Can you work these out from the model? Positions are in its coordinate system, mm. A direction names the side the tool comes from. Give positions to 0.01 mm unless a question says otherwise; leave off trailing zeros. Loops run counter-clockwise (first coordinate to the right, second up) from the corner with the lowest first, then second, coordinate; pieces in that order, holes last. Notation, with made-up numbers: (25.25, 80) - (51.25, 80) arc R24 cw to (51.25, 95) - close; hole circle Ø6 at (-4, -37.75). An arc over 180 degrees is marked (long way). Answer in a Markdown table with one row per item.
from build123d import *

# Parameters (mm, degrees)
SKETCH_1_W                       = 50
SKETCH_1_H                       = 20
SM_BASE_FLANGE_1_DEPTH           = 2
SM_EDGE_FLANGE_1_STRIP_W         = 9.4732
SM_EDGE_FLANGE_1_STRIP_H         = 2
SM_EDGE_FLANGE_1_STRIP_CUT_DEPTH = 20
SM_EDGE_FLANGE_1_DEPTH           = 20
SM_EDGE_FLANGE_2_STRIP_W         = 9.4732
SM_EDGE_FLANGE_2_STRIP_H         = 2
SM_EDGE_FLANGE_2_STRIP_CUT_DEPTH = 20
SM_EDGE_FLANGE_2_DEPTH           = 20
SKETCH_12_R                      = 2
CUT_EXTRUDE_1_DEPTH              = 2
CUT_EXTRUDE_2_REACH              = 61.372
SKETCH_13_R                      = 2


# Sheet-metal steps are written as plain solids
with BuildPart() as part:
    # Sketch 1 → Базовая кромка1 (new body)
    with BuildSketch(Plane(origin=(0, 0, 0), x_dir=(1, 0, 0), z_dir=(0, 1, 0))):
        with Locations((25, 10)):
            Rectangle(SKETCH_1_W, SKETCH_1_H)
    extrude(amount=-SM_BASE_FLANGE_1_DEPTH)

    # Ребро-кромка1 strip (across the edge) → Ребро-кромка1 strip cut (cut)
    with BuildSketch(Plane(origin=(50, 0, 0), x_dir=(-1, 0, 0), z_dir=(0, 0, -1))):
        with Locations((-2, -1)):
            Rectangle(SM_EDGE_FLANGE_1_STRIP_W, SM_EDGE_FLANGE_1_STRIP_H)
    extrude(amount=SM_EDGE_FLANGE_1_STRIP_CUT_DEPTH, mode=Mode.SUBTRACT)

    # Ребро-кромка1 section (across the edge) → Ребро-кромка1 (add)
    with BuildSketch(Plane(origin=(50, 0, 0), x_dir=(-1, 0, 0), z_dir=(0, 0, -1))):
        with BuildLine():
            Line((0, 0.7366), (0, 25))
            Line((0, 25), (2, 25))
            Line((2, 25), (2, 0.7366))
            ThreePointArc((2, 0.7366), (2.215745145, 0.215745145), (2.7366, 0))
            Line((2.7366, 0), (2.7366, -2))
            ThreePointArc((2.7366, -2), (0.801531583, -1.198468417), (0, 0.7366))
        make_face()
    extrude(amount=SM_EDGE_FLANGE_1_DEPTH)

    # Ребро-кромка2 strip (across the edge) → Ребро-кромка2 strip cut (cut)
    with BuildSketch(Plane.XY.offset(-20)):
        with Locations((-2, -1)):
            Rectangle(SM_EDGE_FLANGE_2_STRIP_W, SM_EDGE_FLANGE_2_STRIP_H)
    extrude(amount=SM_EDGE_FLANGE_2_STRIP_CUT_DEPTH, mode=Mode.SUBTRACT)

    # Ребро-кромка2 section (across the edge) → Ребро-кромка2 (add)
    with BuildSketch(Plane.XY.offset(-20)):
        with BuildLine():
            Line((0, 0.7366), (0, 25))
            Line((0, 25), (2, 25))
            Line((2, 25), (2, 0.7366))
            ThreePointArc((2, 0.7366), (2.215745145, 0.215745145), (2.7366, 0))
            Line((2.7366, 0), (2.7366, -2))
            ThreePointArc((2.7366, -2), (0.801531583, -1.198468417), (0, 0.7366))
        make_face()
    extrude(amount=SM_EDGE_FLANGE_2_DEPTH)

    # Эскиз12 → Вырез-Вытянуть1 (cut)
    with BuildSketch(Plane.XZ.offset(2)):
        with Locations(Location((25, -5, 0), (0, 0, 270))):
            Circle(SKETCH_12_R)
        with Locations(Location((25, -15, 0), (0, 0, 270))):
            Circle(SKETCH_12_R)
    extrude(amount=-CUT_EXTRUDE_1_DEPTH, mode=Mode.SUBTRACT)

    # Вырез-Вытянуть2: up to this face of the body (flat: up to its plane)
    cut_extrude_2_end = Plane(part.part.faces().sort_by_distance((0, 12.8683, -10))[0])
    # Эскиз13 → Вырез-Вытянуть2 (cut, up to the picked face)
    with BuildSketch(Plane(origin=(50, 0, 0), x_dir=(0, 0, -1), z_dir=(1, 0, 0)), mode=Mode.PRIVATE) as cut_extrude_2_sk1:
        with Locations(Location((10, 8, 0), (0, 0, 90))):
            Circle(SKETCH_13_R)
    cut_extrude_2_tool1 = split(extrude(cut_extrude_2_sk1.sketch, amount=-CUT_EXTRUDE_2_REACH, mode=Mode.PRIVATE), bisect_by=cut_extrude_2_end, keep=Keep.BOTH, mode=Mode.PRIVATE)
    # Эскиз13 → Вырез-Вытянуть2 (cut, up to the picked face)
    with BuildSketch(Plane(origin=(50, 0, 0), x_dir=(0, 0, -1), z_dir=(1, 0, 0)), mode=Mode.PRIVATE) as cut_extrude_2_sk2:
        with Locations(Location((10, 18, 0), (0, 0, 90))):
            Circle(SKETCH_13_R)
    cut_extrude_2_tool2 = split(extrude(cut_extrude_2_sk2.sketch, amount=-CUT_EXTRUDE_2_REACH, mode=Mode.PRIVATE), bisect_by=cut_extrude_2_end, keep=Keep.BOTH, mode=Mode.PRIVATE)
    add(cut_extrude_2_tool1.solids().sort_by(Axis((50, 8, -10), (-1, 0, 0)))[0], mode=Mode.SUBTRACT)
    add(cut_extrude_2_tool2.solids().sort_by(Axis((50, 18, -10), (-1, 0, 0)))[0], mode=Mode.SUBTRACT)


solid = part.part
Q1. Imagine slicing it at B-B, the plane z = -10. Write out the boundary of the cut face in (x, y), and give its area (3 significant figures).
Checked values:
| item | result |
|---|---|
| outline | (0, 0.74) arc R2.74 ccw to (2.74, -2) - (47.26, -2) arc R2.74 ccw to (50, 0.74) - (50, 6) - (48, 6) - (48, 0.74) arc R0.74 cw to (47.26, 0) - (2.74, 0) arc R0.74 cw to (2, 0.74) - (2, 6) - (0, 6) - close; (0, 10) - (2, 10) - (2, 16) - (0, 16) - close; (0, 20) - (2, 20) - (2, 25) - (0, 25) - close; (48, 10) - (50, 10) - (50, 16) - (48, 16) - close; (48, 20) - (50, 20) - (50, 25) - (48, 25) - close |
| area | 165 mm² |
Q2. Imagine slicing it at C-C, the plane z = -5. Write out the boundary of the cut face in (x, y).
Checked values:
| item | result |
|---|---|
| outline | (0, 0.74) arc R2.74 ccw to (2.74, -2) - (23, -2) - (23, 0) - (2.74, 0) arc R0.74 cw to (2, 0.74) - (2, 25) - (0, 25) - close; (27, -2) - (47.26, -2) arc R2.74 ccw to (50, 0.74) - (50, 25) - (48, 25) - (48, 0.74) arc R0.74 cw to (47.26, 0) - (27, 0) - close |
Q3. If we mould it in two halves opening along Z, with no side actions, what happens to faces 1 (the face through (23, -1, -15)), 2 (the face through (1.014, 16.526, -8.648)), 3 (the face through (25.1, -0.4, -20)), 4 (the face through (49.177, -1.22, -9.86))? For each: released by +Z, released by -Z, zero draft, split by the parting line, or undercut.
Checked values:
| item | result |
|---|---|
| face 1 | undercut |
| face 2 | undercut |
| face 3 | released by -Z |
| face 4 | zero draft |
Q4. If I drill on line 1 (X direction, y = 8.25, z = -12.25); line 2 (Z direction, x = 0.9, y = 8); line 3 (Y direction, x = 12, z = -14.5), over which ranges is the centre line in solid material (lowest first)? Write a range as [from, to].
Checked values:
| item | result |
|---|---|
| line 1 | x = [0, 2], [48, 50] |
| line 2 | z = [-20, -12], [-8, 0] |
| line 3 | y = [-2, 0] |
Q5. On a 3-axis mill with a long thin cutter (end or side, diameter ignored), from which of +Z, -Z, +X, -X, +Y, -Y can I reach the whole of each face in a straight line? I mean faces 5 (the face through (25, 0, -10)), 6 (the face through (0, 13, -10)). Say none if no direction works.
Checked values:
| item | result |
|---|---|
| face 5 | +Z, -Z, +Y |
| face 6 | +Z, -Z, -X, +Y, -Y |
Q6. Imagine slicing it at D-D, the plane y = 8. Write out the boundary of the cut face in (x, z).
Checked values:
| item | result |
|---|---|
| outline | (0, -20) - (2, -20) - (2, -12) - (0, -12) - close; (0, -8) - (2, -8) - (2, 0) - (0, 0) - close; (48, -20) - (50, -20) - (50, -12) - (48, -12) - close; (48, -8) - (50, -8) - (50, 0) - (48, 0) - close |
Q7. Imagine slicing it at A-A, the plane y = 11.5. Write out the boundary of the cut face in (x, z), and give its area (3 significant figures).
Checked values:
| item | result |
|---|---|
| outline | (0, -20) - (2, -20) - (2, 0) - (0, 0) - close; (48, -20) - (50, -20) - (50, 0) - (48, 0) - close |
| area | 80.0 mm² |
Q8. For pin 1 (3.5 mm diameter, centred on y = 18, z = -10, fed in from +X); pin 2 (8 mm diameter, centred on x = 28.5, z = -5.5, fed in from +Y), each with a flat end and sliding along its axis, tell me the tip position at first contact or that it passes through.
Checked values:
| item | result |
|---|---|
| pin 1 | passes through |
| pin 2 | stops at y = 0 |
